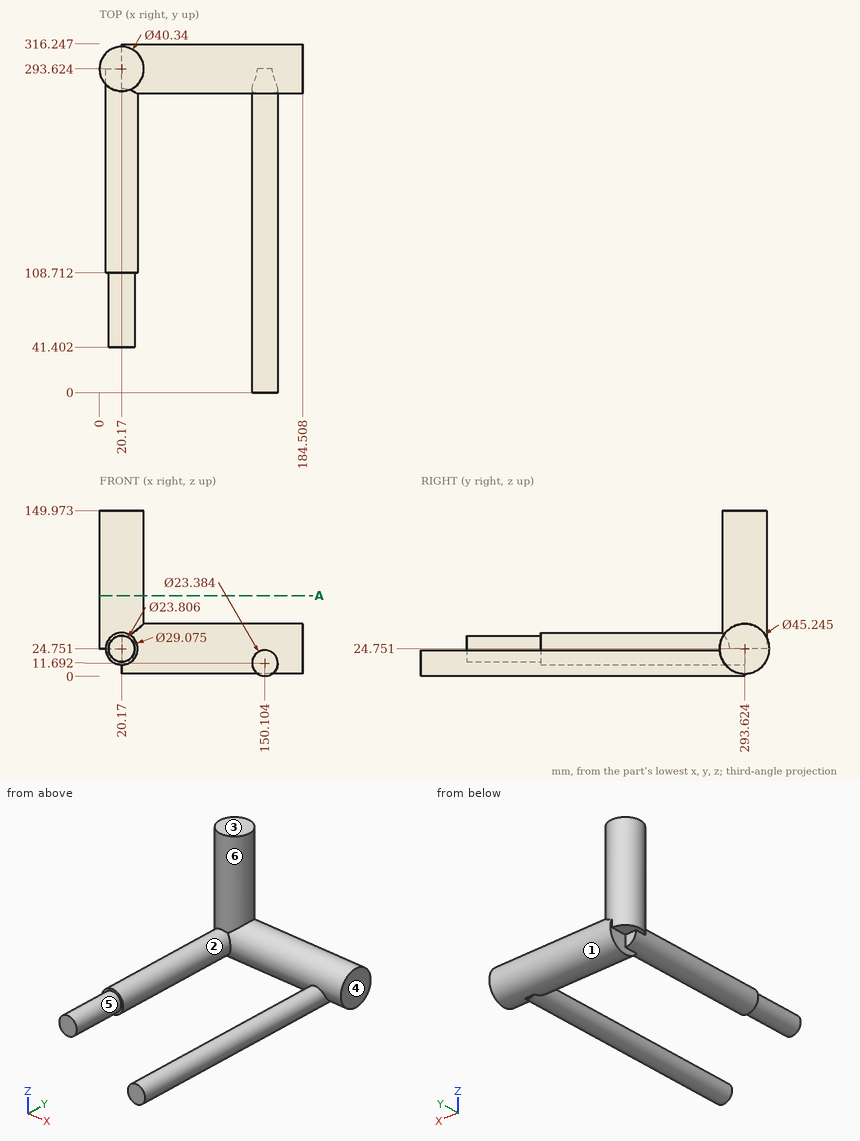
Verification items for this drawing (mm, ordinates from the low corner). A direction names the side the tool comes from. Coordinates: 2 decimals unless noted, no trailing zeros. Order: outer loops, then holes, each group sorted by start corner. A loop starts at its lowest first (then second) coordinate and runs counter-clockwise, first axis right, second up. Notation, with made-up numbers: (30.25, -6) - (39.25, -6) arc R30 ccw to (39.25, 18) - close; hole circle Ø6 at (1, 23.25). An arc over 180 degrees is marked (long way). Answer in a Markdown table with one row per item. Add a question column.
1. Draft check along X on the marked faces 3, 4, 5 and 6. Enter one of: +X half, -X half, draft (parallel to the pull), parting line (faces both ways), or undercut.
2. Material ranges on L1, parallel to X at y = 166, z = 24.5 (1 decimal); L2, parallel to X at y = 227, z = 22.5 (1 decimal); L3, parallel to X at y = 296, z = 34.5, recorded low to high. Write a range as [from, to].
3. Gauge pin test, flat ends, axial feed: pin 1 Ø11.5 at (x, z) = (10.5, 16.5) entering from +Y; pin 2 Ø10 at (y, z) = (289.5, 14) entering from -X; pin 3 Ø1.5 at (x, z) = (101.5, 43.5) entering from -Y. Record the tip position at first contact, or that the pin passes through.
4. Access from +Z, -Z, +X, -X, +Y, -Y to the whole of each face (thin tool, end or side, straight path). Record for the marked faces 1 and 2.
5. Section check A-A (z = 73). Enter the section's corners in (x, y), plus the area to 3 significant figures.
Data:
| question | item | result |
|---|---|---|
| 1 | face 3 | draft |
| 1 | face 4 | +X half |
| 1 | face 5 | undercut |
| 1 | face 6 | parting line |
| 2 | L1 | x = [5.6, 34.7] |
| 2 | L2 | x = [5.8, 34.5], [145.6, 154.6] |
| 2 | L3 | x = [0.14, 184.51] |
| 3 | pin 1 | stops at y = 293.62 |
| 3 | pin 2 | stops at x = 6.82 |
| 3 | pin 3 | stops at y = 279.92 |
| 4 | face 1 | none |
| 4 | face 2 | -Y |
| 5 | outline | circle Ø40.34 at (20.17, 293.62) |
| 5 | area | 1,280 mm² |
